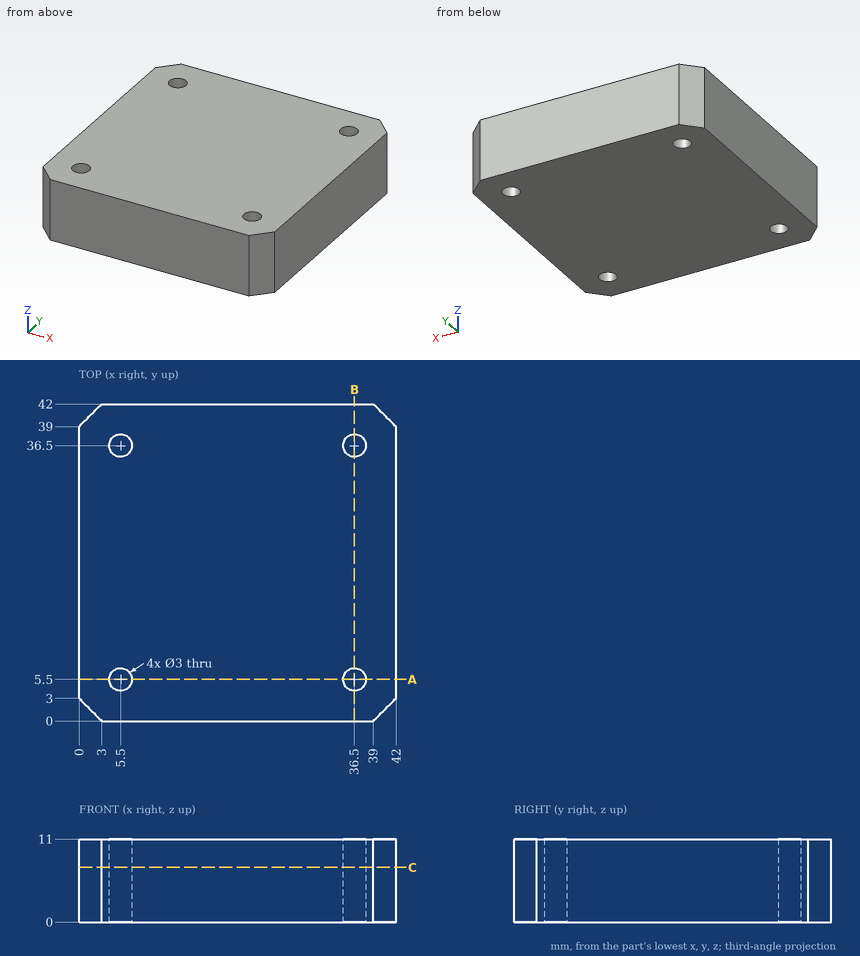
Source: three-view drawing plus pictorial views. Frame: mm from the lowest corner of the part. Give positions to 0.01 mm unless a question says otherwise; leave off trailing zeros. Write each loop counter-clockwise with the first axis right and the second up, starting at its lowest first coordinate (ties: lowest second). Pieces come first, ordered by that corner, then holes. Notation, with made-up numbers: (14, -8) -> (50, -8) arc R23 ccw to (50, 13) -> close; hole circle Ø3 at (86.5, 66.5). An arc over 180 degrees is marked (long way). Write item = value, one per line.
Q1. Cut plane C-C on z = 7.25. Return loops of the section in (x, y).
Here are the results:
outline = (0, 3) -> (3, 0) -> (39, 0) -> (42, 3) -> (42, 39) -> (39, 42) -> (3, 42) -> (0, 39) -> close; hole circle Ø3 at (5.5, 5.5); hole circle Ø3 at (5.5, 36.5); hole circle Ø3 at (36.5, 5.5); hole circle Ø3 at (36.5, 36.5)
Q2. Line query: line 1 (Y direction, x = 5.5, z = 8); line 2 (Y direction, x = 37, z = 3.5). Output: solid intervals per line, ascending. Write a range as from..to.
Here are the results:
line_1 = 0..4, 7..35, 38..42
line_2 = 0..4.09, 6.91..35.09, 37.91..42
Q3. Cut plane A-A on y = 5.5. Return loops of the section in (x, z), then the cut area to 3 significant figures.
Here are the results:
outline = (0, 0) -> (4, 0) -> (4, 11) -> (0, 11) -> close; (7, 0) -> (35, 0) -> (35, 11) -> (7, 11) -> close; (38, 0) -> (42, 0) -> (42, 11) -> (38, 11) -> close
area = 396 mm²
